```python
from build123d import *

# Parameters (mm, degrees)
EXTRUDE_1_DEPTH = 2
SKETCH_2_R      = 4
EXTRUDE_2_DEPTH = 6.5
SKETCH_3_R      = 1.5
EXTRUDE_3_DEPTH = 10.5


with BuildPart() as part:
    # 草图1 → 凸台-拉伸1 (new body)
    with BuildSketch(Plane.XY):
        with BuildLine():
            Line((-4.5, 12), (4.5, 12))
            ThreePointArc((4.5, 12), (9.857189903, 10.7378078), (14.087412587, 7.216752724))
            ThreePointArc((14.087412587, 7.216752724), (16.191153731, 5.146301215), (18.807692308, 3.780203808))
            ThreePointArc((18.807692308, 3.780203808), (21.5, 0), (18.807692308, -3.780203808))
            ThreePointArc((18.807692308, -3.780203808), (16.191153731, -5.146301215), (14.087412587, -7.216752724))
            ThreePointArc((14.087412587, -7.216752724), (9.857189903, -10.7378078), (4.5, -12))
            Line((4.5, -12), (-4.5, -12))
            ThreePointArc((-4.5, -12), (-9.857189903, -10.7378078), (-14.087412587, -7.216752724))
            ThreePointArc((-14.087412587, -7.216752724), (-16.191153731, -5.146301215), (-18.807692308, -3.780203808))
            ThreePointArc((-18.807692308, -3.780203808), (-21.5, 0), (-18.807692308, 3.780203808))
            ThreePointArc((-18.807692308, 3.780203808), (-16.191153731, 5.146301215), (-14.087412587, 7.216752724))
            ThreePointArc((-14.087412587, 7.216752724), (-9.857189903, 10.7378078), (-4.5, 12))
        make_face()
    extrude(amount=-EXTRUDE_1_DEPTH)

    # 草图2 → 凸台-拉伸2 (add)
    with BuildSketch(Plane(origin=(0, 0, -2), x_dir=(-1, 0, 0), z_dir=(0, 0, -1))):
        with Locations(Location((17.5, 0, 0), (0, 0, 289.082124804))):
            Circle(SKETCH_2_R)
        with Locations(Location((-17.5, 0, 0), (0, 0, 250.917875196))):
            Circle(SKETCH_2_R)
    extrude(amount=EXTRUDE_2_DEPTH)

    # 草图3 → 凸台-拉伸3 (add)
    with BuildSketch(Plane(origin=(0, 0, -8.5), x_dir=(-1, 0, 0), z_dir=(0, 0, -1))):
        with Locations(Location((17.5, 0, 0), (0, 0, 180))):
            Circle(SKETCH_3_R)
        with Locations(Location((-17.5, 0, 0), (0, 0, 180))):
            Circle(SKETCH_3_R)
    extrude(amount=EXTRUDE_3_DEPTH)


solid = part.part
```
Geometry: final body of the model. Coordinates: model frame, mm. A direction names the side the tool comes from. Coordinates: 2 decimals unless noted, no trailing zeros. Order: outer loops, then holes, each group sorted by start corner. A loop starts at its lowest first (then second) coordinate and runs counter-clockwise, first axis right, second up. Notation, with made-up numbers: (-10.5, -26) -> (29.5, -26) arc R15 cw to (29.5, 3) -> close; hole circle Ø2 at (84.25, 49.5). An arc over 180 degrees is marked (long way). Answer in a Markdown table with one row per item.
Item 1: Draft query along X for faces 1 (the flat face through (0, 12, -1)), 2 (the cylindrical face through (16, 0, -14)), 3 (the cylindrical face through (-16.16, -5.17, -0.99)). Return one class per face: released by +X, released by -X, zero draft, split by the parting line, or undercut.
Return value:
| item | result |
|---|---|
| face 1 | zero draft |
| face 2 | undercut |
| face 3 | released by -X |
Item 2: Ray query, L1, parallel to Z at x = -1.5, y = -6.25; L2, parallel to X at y = -1.75, z = -6; L3, parallel to Y at x = -14, z = -1.75. Return the intervals inside material, ascending.
Return value:
| item | result |
|---|---|
| L1 | z = -2 to 0 |
| L2 | x = -21.1 to -13.9, 13.9 to 21.1 |
| L3 | y = -7.33 to 7.33 |
Item 3: Access query for faces 4 (the flat face through (-18, -2, -8.5)), 5 (the cylindrical face through (9.93, -10.7, -0.99)). Directions: +Z, -Z, +X, -X, +Y, -Y. A direction counts if a zero-diameter tool reaches every point of the face in a straight line with its end or side. Return the directions, or none.
Return value:
| item | result |
|---|---|
| face 4 | -Z |
| face 5 | +Z, -Z, +X, -Y |
Item 4: Section D-D on z = -11.25. Output: boundary loops of the cut face in (x, y), plus the area to 3 significant figures.
Return value:
| item | result |
|---|---|
| outline | circle Ø3 at (-17.5, 0); circle Ø3 at (17.5, 0) |
| area | 14.1 mm² |
Item 5: Section A-A on z = -8. Output: boundary loops of the cut face in (x, y).
Return value:
| item | result |
|---|---|
| outline | circle Ø8 at (-17.5, 0); circle Ø8 at (17.5, 0) |
Item 6: Section B-B on x = 17.5. Output: boundary loops of the cut face in (y, z).
Return value:
| item | result |
|---|---|
| outline | (-4.34, -2) -> (-4, -2) -> (-4, -8.5) -> (-1.5, -8.5) -> (-1.5, -19) -> (1.5, -19) -> (1.5, -8.5) -> (4, -8.5) -> (4, -2) -> (4.34, -2) -> (4.34, 0) -> (-4.34, 0) -> close |
Item 7: Section C-C on y = 4.5. Output: boundary loops of the cut face in (x, z).
Return value:
| item | result |
|---|---|
| outline | (-17.2, -2) -> (17.2, -2) -> (17.2, 0) -> (-17.2, 0) -> close |
Item 8: Contact query for flat-ended pins moving along their axis: P1, Ø5, axis at x = -1, y = 6.5, coming from the -Z side; P2, Ø12, axis at x = -13.5, y = -8, coming from the -Z side. Output: stop coordinate, or through.
Return value:
| item | result |
|---|---|
| P1 | stops at z = -2 |
| P2 | stops at z = -8.5 |
